Read the model definition and answer for the solid it produces. Units are mm, in the model's axes. Give positions to 0.01 mm unless a question says otherwise; leave off trailing zeros. Write each loop counter-clockwise with the first axis right and the second up, starting at its lowest first coordinate (ties: lowest second). Pieces come first, ordered by that corner, then holes.
Autodesk Inventor part; units mm, degrees
ref_plane "YZ Plane" through (0, 0, 0) normal (1, 0, 0) x (0, 1, 0)
ref_plane "XZ Plane" through (0, 0, 0) normal (0, 1, 0) x (-1, 0, 0)
ref_plane "XY Plane" through (0, 0, 0) normal (0, 0, 1) x (1, 0, 0)
sketch "Sketch1" plane through (0, 0, 0) normal (0, 0, 1) x (1, 0, 0)
  line L0 (-0.6632, 1.4381) -> (-3.6858, 1.4381)
  line L1 (-3.6858, 1.4381) -> (-3.6858, 3.9781)
  line L2 (-3.6858, 3.9781) -> (-0.6632, 3.9781)
  line L3 (-0.6632, 3.9781) -> (-0.6632, 1.4381)
  dimension "d0" = 3.0226
  dimension "d1" = 2.54
extrude "Extrusion1" add sketch "Sketch1" along normal blind 1.27
sketch "Sketch2" plane through (0, 0, 1.27) normal (0, 0, 1) x (1, 0, 0)
  line L0 (-2.5047, 3.0383) -> (-1.8443, 3.0383)
  line L1 (-1.8443, 3.0383) -> (-1.8443, 2.3779)
  line L2 (-1.8443, 2.3779) -> (-2.5047, 2.3779)
  line L3 (-2.5047, 2.3779) -> (-2.5047, 3.0383)
  point P0 (-2.1745, 2.7081)
  dimension "d6" = 0.3302
  dimension "d7" = 0.3302
  dimension "d8" = 0.3302
  dimension "d9" = 0.3302
extrude "Extrusion2" add sketch "Sketch2" along normal blind 6.096
fillet "Fillet1" radius 0.254 4 edges at (-2.1745, 2.3779, 7.366) (-1.8443, 2.7081, 7.366) (-2.1745, 3.0383, 7.366) (-2.5047, 2.7081, 7.366)
fillet "Fillet2" radius 0.254 4 edges at (-3.6858, 1.4381, 0.635) (-0.6632, 1.4381, 0.635) (-0.6632, 3.9781, 0.635) (-3.6858, 3.9781, 0.635)
properties part number "2009_CTS_CopperPost"
Item 1: Each of these flat-tipped pins is pushed along its axis until it touches: pin 1 Ø1 at (y, z) = (3, 3.5) entering from -X; pin 2 Ø1 at (x, z) = (-1.5, 2.5) entering from -Y; pin 3 Ø1.5 at (x, z) = (-3, 4.5) entering from +Y; pin 4 Ø1 at (x, z) = (-3.5, 2) entering from -Y. Where does it stop, or does it pass through?
Result set:
pin 1: stops at x = -2.5
pin 2: stops at y = 2.38
pin 3: stops at y = 3.04
pin 4: passes through
Item 2: Section B-B (x = -2.8) is taken. Write down the section's boundary in (y, z), and give its area (3 significant figures).
Result set:
outline: (1.44, 0) - (3.98, 0) - (3.98, 1.27) - (1.44, 1.27) - close
area: 3.23 mm2
Item 3: Section A-A (y = 2.5) is taken. Write down the section's boundary in (x, z).
Result set:
outline: (-3.69, 0) - (-0.66, 0) - (-0.66, 1.27) - (-1.84, 1.27) - (-1.84, 7.11) arc R0.25 ccw to (-1.97, 7.33) - (-2.38, 7.33) arc R0.25 ccw to (-2.5, 7.11) - (-2.5, 1.27) - (-3.69, 1.27) - close
Item 4: Section C-C (z = 4.5) is taken. Write down the section's boundary in (x, y), and give its area (3 significant figures).
Result set:
outline: (-2.5, 2.38) - (-1.84, 2.38) - (-1.84, 3.04) - (-2.5, 3.04) - close
area: 0.436 mm2
Item 5: Find the intervals of material crossed by line 1 along Z through (x, y) = (-0.9, 1.8); line 2 along Y through (x, z) = (-1.9, 6.5); line 3 along Y through (x, z) = (-3.5, 1), in increasing order.
Result set:
line 1: z = 0 to 1.27
line 2: y = 2.38 to 3.04
line 3: y = 1.45 to 3.97
Item 6: Determine the mould class of faces 1 (the flat face through (-2, 3, 0)), 2 (the flat face through (-2, 1.438, 1)), 3 (the flat face through (-2, 3.978, 1)) for opening direction Y: pulls with the +Y half, pulls with the -Y half, needs draft (parallel to the pull), parting line crosses it, or undercut.
Result set:
face 1: needs draft
face 2: pulls with the -Y half
face 3: pulls with the +Y half
